```python
from build123d import *

# Parameters (mm, degrees)
SKETCH1_W                      = 12.7
SKETCH1_H                      = 323.5
BOSS_EXTRUDE1_DEPTH            = 1.5875
SKETCH2_W                      = 1.5875
SKETCH2_H                      = 323.5
BOSS_EXTRUDE2_DEPTH            = 11.1125
FILLET1_R                      = 1
M2_CLEARANCE_HOLE1_D           = 2.4
M2_CLEARANCE_HOLE1_DEPTH       = 2
M2_CLEARANCE_HOLE1_CSINK_D     = 4.6
M2_CLEARANCE_HOLE1_CSINK_ANGLE = 90
M2_CLEARANCE_HOLE1_TIP         = 0.721032743
M2_CLEARANCE_HOLE2_D           = 2.4
M2_CLEARANCE_HOLE2_DEPTH       = 2
M2_CLEARANCE_HOLE2_CSINK_D     = 4.6
M2_CLEARANCE_HOLE2_CSINK_ANGLE = 90
M2_CLEARANCE_HOLE2_TIP         = 0.721032743


with BuildPart() as part:
    # Sketch1 → Boss-Extrude1 (new body)
    with BuildSketch(Plane(origin=(0, 0, 0), x_dir=(1, 0, 0), z_dir=(0, 1, 0))):
        with Locations((6.35, -161.75)):
            Rectangle(SKETCH1_W, SKETCH1_H)
    extrude(amount=BOSS_EXTRUDE1_DEPTH)

    # Sketch2 → Boss-Extrude2 (add)
    with BuildSketch(Plane(origin=(0, 1.5875, 0), x_dir=(1, 0, 0), z_dir=(0, 1, 0))):
        with Locations((0.79375, -161.75)):
            Rectangle(SKETCH2_W, SKETCH2_H)
    extrude(amount=BOSS_EXTRUDE2_DEPTH)

    # Fillet1
    fillet1_edges = [part.edges().sort_by_distance(p)[0] for p in [
        (0, 0, 161.75),
    ]]
    fillet(fillet1_edges, radius=FILLET1_R)

    # M2 Clearance Hole1
    with Locations(Plane.ZY):
        with Locations((4, 9.5875), (12, 9.5875), (139.3, 9.5875), (206.3, 9.5875), (319.5, 9.5875), (311.5, 9.5875)):
            CounterSinkHole(M2_CLEARANCE_HOLE1_D / 2, M2_CLEARANCE_HOLE1_CSINK_D / 2, depth=M2_CLEARANCE_HOLE1_DEPTH, counter_sink_angle=M2_CLEARANCE_HOLE1_CSINK_ANGLE)
            with Locations((0, 0, -(M2_CLEARANCE_HOLE1_DEPTH + M2_CLEARANCE_HOLE1_TIP / 2))):  # 118° drill point
                Cone(0, M2_CLEARANCE_HOLE1_D / 2, M2_CLEARANCE_HOLE1_TIP, mode=Mode.SUBTRACT)

    # M2 Clearance Hole2
    with Locations(Plane(origin=(0, 0, 0), x_dir=(-1, 0, 0), z_dir=(0, -1, 0))):
        with Locations((-9.5875, -4), (-9.5875, -12), (-9.5875, -139.3), (-9.5875, -206.3), (-9.5875, -311.5), (-9.5875, -319.5)):
            CounterSinkHole(M2_CLEARANCE_HOLE2_D / 2, M2_CLEARANCE_HOLE2_CSINK_D / 2, depth=M2_CLEARANCE_HOLE2_DEPTH, counter_sink_angle=M2_CLEARANCE_HOLE2_CSINK_ANGLE)
            with Locations((0, 0, -(M2_CLEARANCE_HOLE2_DEPTH + M2_CLEARANCE_HOLE2_TIP / 2))):  # 118° drill point
                Cone(0, M2_CLEARANCE_HOLE2_D / 2, M2_CLEARANCE_HOLE2_TIP, mode=Mode.SUBTRACT)


solid = part.part
```
CAD build for the part. Positions are in the model's coordinates, mm. A direction names the side the tool comes from. Round coordinates to 2 decimals unless told otherwise and drop trailing zeros. Loops run counter-clockwise (first coordinate to the right, second up) from the corner with the lowest first, then second, coordinate; pieces in that order, holes last. Notation, with made-up numbers: M 15,-0.5 L 72,-0.5 A27 cw 72,30.5 Z; hole C 14.5,27.25 d5. An arc over 180 degrees is marked long. Use a Markdown table: item, result. Add a question column.
(1) Cut at B-B (x = 4). Give the cut face in (y, z).
(2) Which spindle directions (+Z, -Z, +X, -X, +Y, -Y) get a long thin tool onto all of the face, cutting with end or side? Do faces 1 (the face through (7, 0, 159)), 2 (the face through (1.588, 7, 164)). Say none if no direction does.
(3) Drill centre lines: line 1 (X direction, y = 1.3, z = 319.5); line 2 (X direction, y = 9.5, z = 217). Where is each one in solid material? Low to high.
(4) Flat gauge pins, fed straight in: pin 1 (4 mm diameter, centred on x = 9.59, z = 319.5, fed in from -Y); pin 2 (1 mm diameter, centred on y = 10, z = 238.5, fed in from -X); pin 3 (3.5 mm diameter, centred on y = 8, z = 155.5, fed in from +X); pin 4 (3 mm diameter, centred on y = 9.59, z = 139.3, fed in from -X). Where does each tip first touch, or does it go through?
(5) Cut at A-A (z = 194). Give the cut face in (x, y).
Geometry says:
| question | item | result |
|---|---|---|
| 1 | outline | M 0,0 L 1.59,0 L 1.59,323.5 L 0,323.5 Z |
| 2 | face 1 | +Z, -Z, +X, -X, -Y |
| 2 | face 2 | +Z, -Z, +X, +Y |
| 3 | line 1 | x = 0 to 8.39, 10.79 to 12.7 |
| 3 | line 2 | x = 0 to 1.59 |
| 4 | pin 1 | stops at y = 0.3 |
| 4 | pin 2 | stops at x = 0 |
| 4 | pin 3 | stops at x = 1.59 |
| 4 | pin 4 | stops at x = 0.8 |
| 5 | outline | M 0,1 A1 ccw 1,0 L 12.7,0 L 12.7,1.59 L 1.59,1.59 L 1.59,12.7 L 0,12.7 Z |
